Check sheet for the modelled part. Datum: model origin and axes. Units: mm. A direction names the side the tool comes from. Give positions to 0.01 mm unless a question says otherwise; leave off trailing zeros. Order: outer loops, then holes, each group sorted by start corner. A loop starts at its lowest first (then second) coordinate and runs counter-clockwise, first axis right, second up.
```python
from build123d import *

# Parameters (mm, degrees)
SKETCH_1_R               = 0.7
SKETCH_1_W               = 25
SKETCH_1_H               = 35
EXTRUDE_1_DEPTH          = 1
SKETCH_3_W               = 27
SKETCH_3_H               = 37
SKETCH_3_W_2             = 25
SKETCH_3_H_2             = 35
EXTRUDE_2_DEPTH          = 20
SKETCH_4_W               = 27
SKETCH_4_H               = 37
EXTRUDE_3_DEPTH          = 1
CUT_EXTRUDE_1_DEPTH      = 37.006943775
CUT_EXTRUDE_1_DEPTH_BACK = 37.006943775
SKETCH_5_W               = 25.000009511
SKETCH_5_H               = 7.845312142
SKETCH_6_W               = 27.00004857
SKETCH_6_H               = 0.999781596
EXTRUDE_4_DEPTH          = 5


with BuildPart() as part:
    # 草图1 → 凸台-拉伸1 (new body)
    with BuildSketch(Plane(origin=(0, 0, 0), x_dir=(1, 0, 0), z_dir=(0, 1, 0))):
        Polygon((-13.5, -2), (-13.5, -18.5), (-2, -18.5), (-2, -22.5), (2, -22.5), (2, -18.5), (13.5, -18.5), (13.5, -2), (17.5, -2), (17.5, 2), (13.5, 2), (13.5, 18.5), (2, 18.5), (2, 22.5), (-2, 22.5), (-2, 18.5), (-13.5, 18.5), (-13.5, 2), (-17.5, 2), (-17.5, -2), align=None)
        with Locations(Location((-15.5, 0, 0), (0, 0, 270))):
            Circle(SKETCH_1_R, mode=Mode.SUBTRACT)
        with Locations(Location((15.5, 0, 0), (0, 0, 270))):
            Circle(SKETCH_1_R, mode=Mode.SUBTRACT)
        with Locations(Location((0, 20.5, 0), (0, 0, 270))):
            Circle(SKETCH_1_R, mode=Mode.SUBTRACT)
        with Locations(Location((0, -20.5, 0), (0, 0, 270))):
            Circle(SKETCH_1_R, mode=Mode.SUBTRACT)
        Rectangle(SKETCH_1_W, SKETCH_1_H, mode=Mode.SUBTRACT)
    extrude(amount=EXTRUDE_1_DEPTH)

    # 草图3 → 凸台-拉伸2 (add)
    with BuildSketch(Plane(origin=(0, 1, 0), x_dir=(1, 0, 0), z_dir=(0, 1, 0))):
        Rectangle(SKETCH_3_W, SKETCH_3_H)
        Rectangle(SKETCH_3_W_2, SKETCH_3_H_2, mode=Mode.SUBTRACT)
    extrude(amount=EXTRUDE_2_DEPTH)

    # 草图4 → 凸台-拉伸3 (add)
    with BuildSketch(Plane(origin=(0, 21, 0), x_dir=(1, 0, 0), z_dir=(0, 1, 0))):
        Rectangle(SKETCH_4_W, SKETCH_4_H)
    extrude(amount=EXTRUDE_3_DEPTH)

    # 草图5 → 切除-拉伸1 (cut, two sides: drawn at the far end of the back side and taken through both)
    with BuildSketch(Plane.XY.offset(-CUT_EXTRUDE_1_DEPTH_BACK)):
        with Locations((2.6183e-05, 17.077384412)):
            Rectangle(SKETCH_5_W, SKETCH_5_H)
    extrude(amount=CUT_EXTRUDE_1_DEPTH + CUT_EXTRUDE_1_DEPTH_BACK, mode=Mode.SUBTRACT)

    # 草图6 → 凸台-拉伸4 (add)
    with BuildSketch(Plane(origin=(0, 0, -18.5), x_dir=(-1, 0, 0), z_dir=(0, 0, -1))):
        with Locations((2.5906e-05, 21.500116927)):
            Rectangle(SKETCH_6_W, SKETCH_6_H)
    extrude(amount=EXTRUDE_4_DEPTH)


solid = part.part
```
(1) Cross-section at D-D on x = -15.5. Enter the section's corners in (y, z), then the cut area to 3 significant figures.
Response values:
outline: (0, -2) - (1, -2) - (1, -0.7) - (0, -0.7) - close; (0, 0.7) - (1, 0.7) - (1, 2) - (0, 2) - close
area: 2.60 mm2
(2) Set-up check for faces 4 (the face through (0, 8, 17.5)), 5 (the face through (-2, 0.5, 20.5)), 6 (the face through (15.5, 0.5, 2)): record each of +Z, -Z, +X, -X, +Y, -Y from which the full face is reachable in a straight line by a thin tool's end or side.
Response values:
face 4: -Y
face 5: +Z, -X, +Y, -Y
face 6: +Z, +X, +Y, -Y
(3) Cross-section at A-A on x = 0. Count the separate pieces of the cut face and the enclosed holes in it, then the cut area to 3 significant figures.
Response values:
separate pieces: 5
enclosed holes: 0
area: 73.5 mm2
(4) Cross-section at B-B on z = -20.5. Enter the section's corners in (x, y).
Response values:
outline: (-13.5, 21) - (13.5, 21) - (13.5, 22) - (-13.5, 22) - close; (-2, 0) - (-0.7, 0) - (-0.7, 1) - (-2, 1) - close; (0.7, 0) - (2, 0) - (2, 1) - (0.7, 1) - close
(5) Release check for a two-part mould opening along Y. For faces 1 (the face through (0, 13.155, -18)), 2 (the face through (-13.5, 11, 0)), 3 (the face through (0, 22, 0)) record: released by +Y, released by -Y, zero draft, split by the parting line, or undercut.
Response values:
face 1: undercut
face 2: zero draft
face 3: released by +Y
(6) Material ranges on L1, parallel to X at y = 0.75, z = 0; L2, parallel to X at y = 17.25, z = 3; L3, parallel to Z at x = 0, y = 9, recorded low to high.
Response values:
L1: x = -17.5 to -16.2, -14.8 to -12.5, 12.5 to 14.8, 16.2 to 17.5
L2: x = -13.5 to -12.5, 12.5 to 13.5
L3: z = -18.5 to -17.5, 17.5 to 18.5
(7) Gauge pin test, flat ends, axial feed: pin 1 Ø0.5 at (x, y) = (16.5, 0.5) entering from -Z; pin 2 Ø4 at (y, z) = (9.5, -6) entering from +X; pin 3 Ø11 at (x, y) = (5.5, 5.5) entering from +Z. Record the tip position at first contact, or that the pin passes through.
Response values:
pin 1: stops at z = -2
pin 2: stops at x = 13.5
pin 3: stops at z = 18.5
